Geometry check sheet. Reference: drawing and pictorial views, mm from the part's lowest x, y, z. Coordinates: 2 decimals unless noted, no trailing zeros. Write each loop counter-clockwise with the first axis right and the second up, starting at its lowest first coordinate (ties: lowest second). Pieces come first, ordered by that corner, then holes. Notation, with made-up numbers: (87, 75) -> (122, 75) arc R5 cw to (122, 82) -> close; hole circle Ø8 at (-23, 62.25). An arc over 180 degrees is marked (long way). Put each result on its own line as item: value.
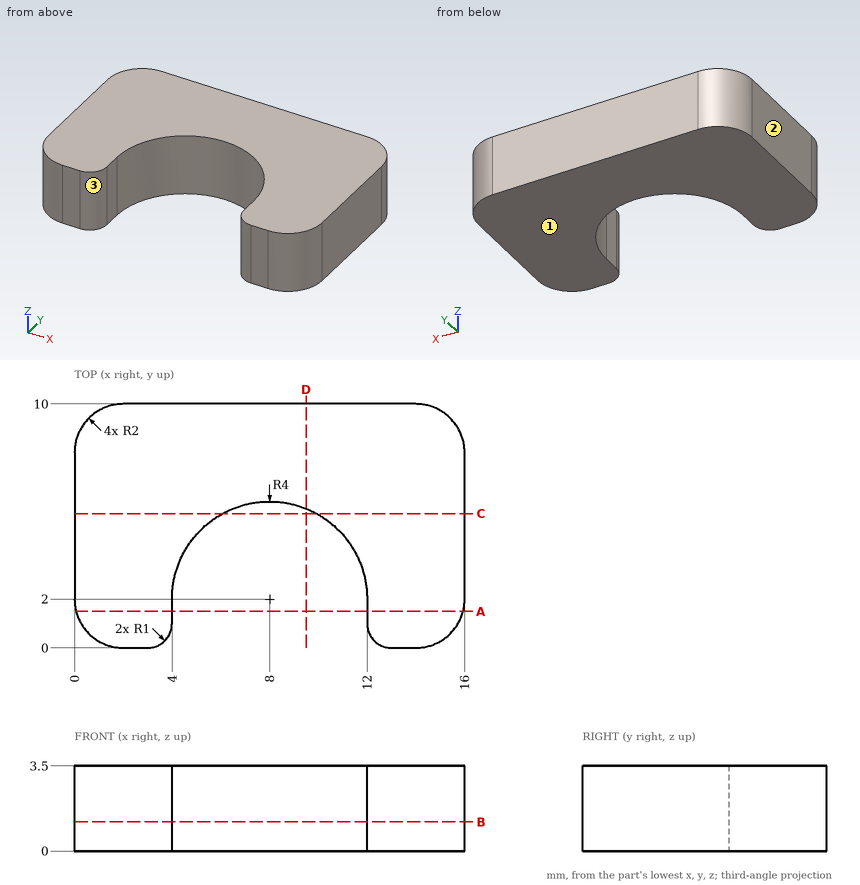
Q1. Cross-section at D-D (x = 9.5). Record the cut outline in (y, z).
Recorded:
outline: (5.71, 0) -> (10, 0) -> (10, 3.5) -> (5.71, 3.5) -> close
Q2. Depth check by flat-ended pin: P1, Ø1, axis at x = 1.5, z = 2.5, coming from the +Y side; P2, Ø0.8, axis at y = 1.5, z = 1, coming from the -X side; P3, Ø1.5, axis at x = 7.5, z = 1.5, coming from the -Y side; P4, Ø0.5, axis at y = 1.5, z = 1, coming from the +X side. Enter the tip coordinate at first touch or a pass-through.
Recorded:
P1: stops at y = 10
P2: stops at x = 0
P3: stops at y = 5.8
P4: stops at x = 15.98
Q3. Cross-section at B-B (z = 1.2). Record the cut outline in (x, y).
Recorded:
outline: (0, 2) arc R2 ccw to (2, 0) -> (3, 0) arc R1 ccw to (4, 1) -> (4, 2) arc R4 cw to (12, 2) -> (12, 1) arc R1 ccw to (13, 0) -> (14, 0) arc R2 ccw to (16, 2) -> (16, 8) arc R2 ccw to (14, 10) -> (2, 10) arc R2 ccw to (0, 8) -> close
Q4. Mould release check, pull along X, two halves, no side actions. Record for the marked faces 1, 2 and 3: released by +X, released by -X, zero draft, split by the parting line, or undercut.
Recorded:
face 1: zero draft
face 2: released by -X
face 3: undercut
Q5. Material ranges on line 1 along X through (y, z) = (2, 1.1); line 2 along X through (y, z) = (3, 1.9); line 3 along Y through (x, z) = (12.75, 3.3), recorded low to high.
Recorded:
line 1: x = 0 to 4, 12 to 16
line 2: x = 0 to 4.13, 11.87 to 16
line 3: y = 0.03 to 10
Q6. Cross-section at A-A (y = 1.5). Record the cut outline in (x, z), plus the area to 3 significant figures.
Recorded:
outline: (0.06, 0) -> (4, 0) -> (4, 3.5) -> (0.06, 3.5) -> close; (12, 0) -> (15.94, 0) -> (15.94, 3.5) -> (12, 3.5) -> close
area: 27.6 mm2
Q7. Cross-section at C-C (y = 5.5). Record the cut outline in (x, z), plus the area to 3 significant figures.
Recorded:
outline: (0, 0) -> (6.06, 0) -> (6.06, 3.5) -> (0, 3.5) -> close; (9.94, 0) -> (16, 0) -> (16, 3.5) -> (9.94, 3.5) -> close
area: 42.4 mm2
